For this review, take the finished solid that the model builds, in its own axes (mm). Face numbers are marked on the shaded views. A direction names the side the tool comes from. Coordinates: 2 decimals unless noted, no trailing zeros. Order: outer loops, then holes, each group sorted by start corner. A loop starts at its lowest first (then second) coordinate and runs counter-clockwise, first axis right, second up. Notation, with made-up numbers: (-3, 43) -> (42, 43) arc R13 ccw to (42, 61) -> close; hole circle Ø10 at (80.25, -22.75). An arc over 180 degrees is marked (long way). Return JSON: item names as keys, results as strings. Group by question number.
Item 1: Take a section at C-C (x = 0). Count the separate pieces of the cut face and the enclosed holes in it, then the cut area to 3 significant figures.
Item 2: Draft analysis for pull direction X (two halves, no side actions). For the marked faces 1, 2 and 3, state which applies: +X half, -X half, draft (parallel to the pull), parting line (faces both ways), or undercut.
Item 3: Machinability: for the marked faces 4, 5 and 6, which of the approach directions +Z, -Z, +X, -X, +Y, -Y give a long, thin tool a straight path to every point of the face, cutting with its end or side? Answer none if there is none.
Item 4: Take a section at D-D (y = 43). Write out the cut boundary in (x, z).
Item 5: Take a section at B-B (z = 0). Write out the cut boundary in (x, y).
Item 6: Insertion check: pin 1 (8 mm diameter, centred on y = 52.5, z = 12.5, fed in from +X); pin 2 (12 mm diameter, centred on x = 5, y = 20.5, fed in from -Z); pin 3 (8 mm diameter, centred on x = -16, z = 4.5, fed in from -Y); pin 4 (22.5 mm diameter, centred on x = 8.5, z = -7, fed in from +Y). Each pin has a flat end and moves straight along its axis. Give the tip position at first contact, or say it passes through.
Item 7: Take a section at A-A (y = 30.48). Write out the cut boundary in (x, z).
Item 8: For line 1 along Y through (x, z) = (18, -9); line 2 along X through (y, z) = (20, 0); line 3 along Y through (x, z) = (0, -18.4), list the stretches that pass through material, from the lowest coordinate up.
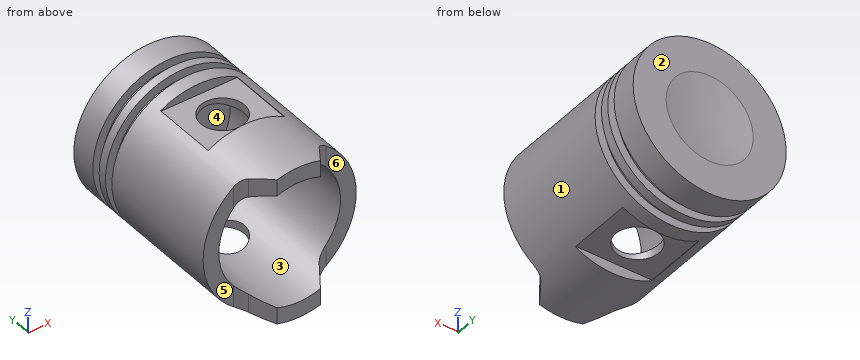
```python
from build123d import *

# Parameters (mm, degrees)
SKETCH3_R               = 17.78
CUT_EXTRUDE2_DEPTH      = 51.816
SKETCH4_R               = 6.35
CUT_EXTRUDE3_DEPTH      = 23.352
CUT_EXTRUDE3_DEPTH_BACK = 23.352
CUT_EXTRUDE5_START      = 19.177
SKETCH5_W               = 22.352
SKETCH5_H               = 19.05
CUT_EXTRUDE5_DEPTH      = 4.1750001
CUT_EXTRUDE6_DEPTH      = 23.352


with BuildPart() as part:
    # Sketch1 → Revolve2 (revolve)
    with BuildSketch(Plane.XY):
        with BuildLine():
            Line((0, 0), (0, 58.166))
            ThreePointArc((0, 58.166), (6.387986381, 58.484288237), (12.712693656, 59.436))
            Line((12.712693656, 59.436), (22.352, 59.436))
            Line((22.352, 59.436), (22.352, 51.816))
            Line((22.352, 51.816), (19.812, 51.816))
            Line((19.812, 51.816), (19.812, 49.276))
            Line((19.812, 49.276), (22.352, 49.276))
            Line((22.352, 49.276), (22.352, 46.736))
            Line((22.352, 46.736), (19.812, 46.736))
            Line((19.812, 46.736), (19.812, 44.196))
            Line((19.812, 44.196), (22.352, 44.196))
            Line((22.352, 44.196), (22.352, 0))
            Line((22.352, 0), (0, 0))
        make_face()
    revolve(axis=Axis((0, 0, 0), (0, 1, 0)))

    # Sketch3 → Cut-Extrude2 (cut)
    with BuildSketch(Plane(origin=(0, 0, 0), x_dir=(-1, 0, 0), z_dir=(0, -1, 0))):
        Circle(SKETCH3_R)
    extrude(amount=-CUT_EXTRUDE2_DEPTH, mode=Mode.SUBTRACT)

    # Sketch4 → Cut-Extrude3 (cut, two sides)
    with BuildSketch(Plane.XY) as cut_extrude3_sk:
        with Locations((0, 30.48)):
            Circle(SKETCH4_R)
    extrude(amount=CUT_EXTRUDE3_DEPTH, mode=Mode.SUBTRACT)
    extrude(cut_extrude3_sk.sketch, amount=-CUT_EXTRUDE3_DEPTH_BACK, mode=Mode.SUBTRACT)

    # Sketch5 → Cut-Extrude5 (cut, through all)
    with BuildSketch(Plane.XY.offset(CUT_EXTRUDE5_START)):
        with Locations((0, 30.48)):
            Rectangle(SKETCH5_W, SKETCH5_H)
    cut_extrude5 = extrude(amount=CUT_EXTRUDE5_DEPTH, mode=Mode.SUBTRACT)

    # Mirror1: Cut-Extrude5 across plane
    add(cut_extrude5.mirror(Plane.XY), mode=Mode.SUBTRACT)

    # Sketch6 → Cut-Extrude6 (cut, symmetric)
    with BuildSketch(Plane.XY):
        with BuildLine():
            Line((22.352, 7.62), (13.470533586, 7.62))
            ThreePointArc((13.470533586, 7.62), (11.673046061, 7.169336035), (10.300788381, 5.923957269))
            Line((10.300788381, 5.923957269), (6.35, 0))
            Line((6.35, 0), (22.352, 0))
            Line((22.352, 0), (22.352, 7.62))
        make_face()
    cut_extrude6 = extrude(amount=CUT_EXTRUDE6_DEPTH, both=True, mode=Mode.SUBTRACT)

    # Mirror2: Cut-Extrude6 across plane
    add(cut_extrude6.mirror(Plane(origin=(0, 0, 0), x_dir=(0, 0, 1), z_dir=(1, 0, 0))), mode=Mode.SUBTRACT)


solid = part.part
```
Findings below:
{
 "1": {"separate pieces": "3", "enclosed holes": "0", "area": "611 mm2"},
 "2": {"face 1": "parting line", "face 2": "draft", "face 3": "undercut"},
 "3": {"face 4": "-Y", "face 5": "+Z, -Z, -X, -Y", "face 6": "+Z, -Z, +X, -Y"},
 "4": {"outline": "circle Ø44.7 at (0, 0); hole circle Ø35.56 at (0, 0)"},
 "5": {"outline": "(-22.35, 7.62) -> (-17.78, 7.62) -> (-17.78, 51.82) -> (17.78, 51.82) -> (17.78, 7.62) -> (22.35, 7.62) -> (22.35, 44.2) -> (19.81, 44.2) -> (19.81, 46.74) -> (22.35, 46.74) -> (22.35, 49.28) -> (19.81, 49.28) -> (19.81, 51.82) -> (22.35, 51.82) -> (22.35, 59.44) -> (12.71, 59.44) arc R64.26 cw to (-12.71, 59.44) -> (-22.35, 59.44) -> (-22.35, 51.82) -> (-19.81, 51.82) -> (-19.81, 49.28) -> (-22.35, 49.28) -> (-22.35, 46.74) -> (-19.81, 46.74) -> (-19.81, 44.2) -> (-22.35, 44.2) -> close"},
 "6": {"pin 1": "stops at x = 20.67", "pin 2": "stops at z = -22.35", "pin 3": "stops at y = 7.62", "pin 4": "stops at y = 59.44"},
 "7": {"outline": "(-11.18, -19.36) -> (-11.18, -19.18) -> (-6.35, -19.18) -> (-6.35, -16.61) arc R17.78 cw to (-6.35, 16.61) -> (-6.35, 19.18) -> (-11.18, 19.18) -> (-11.18, 19.36) arc R22.35 ccw to start; (6.35, -19.18) -> (11.18, -19.18) -> (11.18, -19.36) arc R22.35 ccw to (11.18, 19.36) -> (11.18, 19.18) -> (6.35, 19.18) -> (6.35, 16.61) arc R17.78 cw to (6.35, -16.61) -> close"},
 "8": {"line 1": "y = 7.62 to 44.2, 46.74 to 49.28, 51.82 to 59.44", "line 2": "x = -22.35 to -17.78, 17.78 to 22.35", "line 3": "y = 0 to 24.13, 36.83 to 59.44"}
}
